Geometry: final body of the model. Coordinates: model frame, mm. Face numbers are marked on the shaded views. A direction names the side the tool comes from. Give positions to 0.01 mm unless a question says otherwise; leave off trailing zeros. Order: outer loops, then holes, each group sorted by start corner. A loop starts at its lowest first (then second) coordinate and runs counter-clockwise, first axis right, second up. Notation, with made-up numbers: M 55,85 L 73,85 A22 ccw 73,107 Z; hole C 21.5,-27.75 d1. An arc over 180 degrees is marked long. Write item = value, one per line. Start each with the question number.
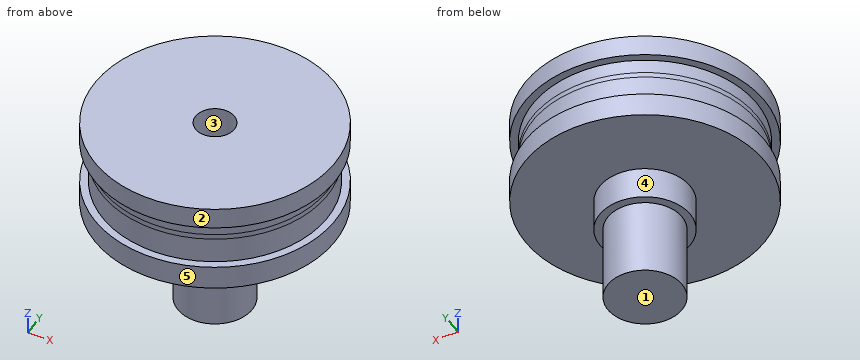
from build123d import *

# Parameters (mm, degrees)
SKETCH_1_R          = 18.5
SKETCH_1_R_2        = 3
EXTRUDE_1_DEPTH     = 14
SKETCH_2_R          = 18.5
SKETCH_2_R_2        = 17.3
CUT_EXTRUDE_1_DEPTH = 2.2
SKETCH_2_2_R        = 18.5
SKETCH_2_2_R_2      = 17.3
CUT_EXTRUDE_2_DEPTH = 0.8
SKETCH_2_4_R        = 18.5
SKETCH_2_4_R_2      = 17.3
CUT_EXTRUDE_3_DEPTH = 4
SKETCH_2_6_R        = 18.5
SKETCH_2_6_R_2      = 17.3
CUT_EXTRUDE_5_DEPTH = 3
SKETCH_3_R          = 7
EXTRUDE_3_DEPTH     = 5
SKETCH_4_R          = 5.75
EXTRUDE_4_DEPTH     = 12


with BuildPart() as part:
    # Sketch 1 → Extrude 1 (new body)
    with BuildSketch(Plane.XY):
        Circle(SKETCH_1_R)
        Circle(SKETCH_1_R_2, mode=Mode.SUBTRACT)
    extrude(amount=EXTRUDE_1_DEPTH)

    # Sketch 2 → Cut-Extrude 1 (cut)
    with BuildSketch(Plane.XY.offset(7.7)):
        Circle(SKETCH_2_R)
        Circle(SKETCH_2_R_2, mode=Mode.SUBTRACT)
    extrude(amount=-CUT_EXTRUDE_1_DEPTH, mode=Mode.SUBTRACT)

    # Sketch 2_2 → Cut-Extrude 2 (cut)
    with BuildSketch(Plane.XY.offset(7.7)):
        Circle(SKETCH_2_2_R)
        Circle(SKETCH_2_2_R_2, mode=Mode.SUBTRACT)
    extrude(amount=CUT_EXTRUDE_2_DEPTH, mode=Mode.SUBTRACT)

    # Sketch 2_4 → Cut-Extrude 3 (cut)
    with BuildSketch(Plane.XY.offset(7.7)):
        Circle(SKETCH_2_4_R)
        Circle(SKETCH_2_4_R_2, mode=Mode.SUBTRACT)
    extrude(amount=-CUT_EXTRUDE_3_DEPTH, mode=Mode.SUBTRACT)

    # Sketch 2_6 → Cut-Extrude 5 (cut)
    with BuildSketch(Plane.XY.offset(7.7)):
        Circle(SKETCH_2_6_R)
        Circle(SKETCH_2_6_R_2, mode=Mode.SUBTRACT)
    extrude(amount=CUT_EXTRUDE_5_DEPTH, mode=Mode.SUBTRACT)

    # Sketch 3 → Extrude 3 (add)
    with BuildSketch(Plane(origin=(0, 0, 0), x_dir=(-1, 0, 0), z_dir=(0, 0, -1))):
        Circle(SKETCH_3_R)
    extrude(amount=EXTRUDE_3_DEPTH)

    # Sketch 4 → Extrude 4 (add)
    with BuildSketch(Plane(origin=(0, 0, -5), x_dir=(-1, 0, 0), z_dir=(0, 0, -1))):
        Circle(SKETCH_4_R)
    extrude(amount=EXTRUDE_4_DEPTH)


solid = part.part
1) Cut plane D-D (x = -10.5). Return loops of the section in (y, z), plus the area to 3 significant figures.
2) Cut plane A-A (x = 0). Return loops of the section in (y, z).
3) Cut plane B-B (y = -11.5). Return loops of the section in (x, z).
4) Ray query, L1, parallel to Z at x = 12, y = -13; L2, parallel to Y at x = 0, z = 3.25; L3, parallel to Y at x = 0, z = 5.75. Return the intervals inside material, ascending.
5) Access query for the marked faces 4 and 5. Directions: +Z, -Z, +X, -X, +Y, -Y. A direction counts if a zero-diameter tool reaches every point of the face in a straight line with its end or side. Return the directions, or none.
6) Pin query (flat end, axial travel): pin 1 Ø1.5 at (y, z) = (-1.5, 8.5) entering from +X; pin 2 Ø10 at (x, z) = (-6.5, 5.5) entering from -Y; pin 3 Ø1 at (y, z) = (8, 7.5) entering from +X. Return the tip coordinate at first contact, or that it passes through.
7) Cut plane C-C (z = 3). Return loops of the section in (x, y), plus the area to 3 significant figures.
8) Draft query along X for the marked faces 1, 2 and 3. Return one class per face: pulls with the +X half, pulls with the -X half, needs draft (parallel to the pull), parting line crosses it, or undercut.
Reply:
q1.outline = M -15.23,0 L 15.23,0 L 15.23,3.7 L 13.75,3.7 L 13.75,10.7 L 15.23,10.7 L 15.23,14 L -15.23,14 L -15.23,10.7 L -13.75,10.7 L -13.75,3.7 L -15.23,3.7 Z
q1.area = 406 mm²
q2.outline = M -18.5,0 L -7,0 L -7,-5 L -5.75,-5 L -5.75,-17 L 5.75,-17 L 5.75,-5 L 7,-5 L 7,0 L 18.5,0 L 18.5,3.7 L 17.3,3.7 L 17.3,10.7 L 18.5,10.7 L 18.5,14 L 3,14 L 3,0 L -3,0 L -3,14 L -18.5,14 L -18.5,10.7 L -17.3,10.7 L -17.3,3.7 L -18.5,3.7 Z
q3.outline = M -14.49,0 L 14.49,0 L 14.49,3.7 L 12.92,3.7 L 12.92,10.7 L 14.49,10.7 L 14.49,14 L -14.49,14 L -14.49,10.7 L -12.92,10.7 L -12.92,3.7 L -14.49,3.7 Z
q4.L1 = 0 to 3.7, 10.7 to 14
q4.L2 = -18.5 to -3, 3 to 18.5
q4.L3 = -17.3 to -3, 3 to 17.3
q5.face_4 = -Z
q5.face_5 = +Z, -Z
q6.pin_1 = 17.28
q6.pin_2 = -18.41
q6.pin_3 = 15.59
q7.outline = C 0,0 d37; hole C 0,0 d6
q7.area = 1,050 mm²
q8.face_1 = needs draft
q8.face_2 = parting line crosses it
q8.face_3 = undercut
